Verification items for the finished model (mm, model axes). A direction names the side the tool comes from. Give positions to 0.01 mm unless a question says otherwise; leave off trailing zeros. Order: outer loops, then holes, each group sorted by start corner. A loop starts at its lowest first (then second) coordinate and runs counter-clockwise, first axis right, second up. Notation, with made-up numbers: (-15, 85) - (5, 85) arc R3 cw to (5, 89) - close; hole circle Ø2 at (-27.75, 44.5). An arc over 180 degrees is marked (long way). Answer as a JSON object with one key per item and string values.
```python
from build123d import *

# Parameters (mm, degrees)
SKETCH1_R           = 50.8
SKETCH1_R_2         = 6.92820323
BOSS_EXTRUDE1_DEPTH = 45.974
SKETCH2_R           = 38.1
CUT_EXTRUDE1_DEPTH  = 25.4


with BuildPart() as part:
    # Sketch1 → Boss-Extrude1 (new body)
    # profile 1 of 7: a face of its own
    with BuildSketch(Plane.XY):
        Circle(SKETCH1_R)
        Circle(SKETCH1_R_2, mode=Mode.SUBTRACT)
    # profile 2 of 7: a face of its own
    with BuildSketch(Plane.XY):
        with BuildLine():
            Line((-3.464101615, -6), (-6.92820323, 0))
            ThreePointArc((-6.92820323, 0), (-6, -3.464101615), (-3.464101615, -6))
        make_face()
    # profile 3 of 7: a face of its own
    with BuildSketch(Plane.XY):
        with BuildLine():
            Line((-6.92820323, 0), (-3.464101615, 6))
            ThreePointArc((-3.464101615, 6), (-6, 3.464101615), (-6.92820323, 0))
        make_face()
    # profile 4 of 7: a face of its own
    with BuildSketch(Plane.XY):
        with BuildLine():
            ThreePointArc((3.464101615, 6), (0, 6.92820323), (-3.464101615, 6))
            Line((-3.464101615, 6), (3.464101615, 6))
        make_face()
    # profile 5 of 7: a face of its own
    with BuildSketch(Plane.XY):
        with BuildLine():
            ThreePointArc((6.92820323, 0), (6, 3.464101615), (3.464101615, 6))
            Line((3.464101615, 6), (6.92820323, 0))
        make_face()
    # profile 6 of 7: a face of its own
    with BuildSketch(Plane.XY):
        with BuildLine():
            ThreePointArc((3.464101615, -6), (6, -3.464101615), (6.92820323, 0))
            Line((6.92820323, 0), (3.464101615, -6))
        make_face()
    # profile 7 of 7: a face of its own
    with BuildSketch(Plane.XY):
        with BuildLine():
            Line((3.464101615, -6), (-3.464101615, -6))
            ThreePointArc((-3.464101615, -6), (0, -6.92820323), (3.464101615, -6))
        make_face()
    extrude(amount=BOSS_EXTRUDE1_DEPTH)

    # Sketch2 → Cut-Extrude1 (cut)
    with BuildSketch(Plane.XY):
        Circle(SKETCH2_R)
    extrude(amount=CUT_EXTRUDE1_DEPTH, mode=Mode.SUBTRACT)


solid = part.part
```
(1) Access from +Z, -Z, +X, -X, +Y, -Y to the whole of each face (thin tool, end or side, straight path). Record for faces 4 (the flat face through (7, 38, 0)), 5 (the flat face through (-5.172, -3.042, 35.543)), 6 (the flat face through (8, 1, 25.4)).
Computed values:
{"face 4": "-Z, +X, -X, +Y, -Y", "face 5": "+Z, -Z", "face 6": "-Z"}
(2) Section check C-C (y = -26.5). Record the cut outline in (x, z).
Computed values:
{"outline": "(-43.34, 0) - (-27.37, 0) - (-27.37, 25.4) - (27.37, 25.4) - (27.37, 0) - (43.34, 0) - (43.34, 45.97) - (-43.34, 45.97) - close"}
(3) Gauge pin test, flat ends, axial feed: pin 1 Ø4 at (x, y) = (-8, 9.5) entering from -Z; pin 2 Ø1.5 at (x, z) = (27, 6) entering from +Y; pin 3 Ø10 at (y, z) = (37, 25.5) entering from +X. Record the tip position at first contact, or that the pin passes through.
Computed values:
{"pin 1": "stops at z = 25.4", "pin 2": "stops at y = 43.49", "pin 3": "stops at x = 39.45"}
(4) Section check B-B (z = 42.5). Record the cut outline in (x, y).
Computed values:
{"outline": "circle Ø101.6 at (0, 0); hole (-6.93, 0) - (-3.46, -6) - (3.46, -6) - (6.93, 0) - (3.46, 6) - (-3.46, 6) - close"}
(5) Section check D-D (x = 32.5). Record the cut outline in (y, z).
Computed values:
{"outline": "(-39.04, 0) - (-19.88, 0) - (-19.88, 25.4) - (19.88, 25.4) - (19.88, 0) - (39.04, 0) - (39.04, 45.97) - (-39.04, 45.97) - close"}
(6) Material ranges on line 1 along Y through (x, z) = (0, 6.5); line 2 along Z through (x, y) = (12, -14.5); line 3 along X through (y, z) = (-1, 12.5), recorded low to high. Write a range as [from, to].
Computed values:
{"line 1": "y = [-50.8, -38.1], [38.1, 50.8]", "line 2": "z = [25.4, 45.97]", "line 3": "x = [-50.79, -38.09], [38.09, 50.79]"}
(7) Release check for a two-part mould opening along Y. For faces 1 (the flat face through (5.22, -2.96, 35.54)), 2 (the flat face through (11, 1, 45.974)), 3 (the cylindrical face through (-11.012, -49.592, 22.665)) record: pulls with the +Y half, pulls with the -Y half, needs draft (parallel to the pull), parting line crosses it, or undercut.
Computed values:
{"face 1": "undercut", "face 2": "needs draft", "face 3": "parting line crosses it"}
(8) Section check A-A (x = 0). Record the cut outline in (y, z), then the cut area to 3 significant figures.
Computed values:
{"outline": "(-50.8, 0) - (-38.1, 0) - (-38.1, 25.4) - (-6, 25.4) - (-6, 45.97) - (-50.8, 45.97) - close; (6, 25.4) - (38.1, 25.4) - (38.1, 0) - (50.8, 0) - (50.8, 45.97) - (6, 45.97) - close", "area": "2,490 mm²"}
